Geometry: final body of the model. Coordinates: model frame, mm. Face numbers are marked on the shaded views. Coordinates: 2 decimals unless noted, no trailing zeros. Write each loop counter-clockwise with the first axis right and the second up, starting at its lowest first coordinate (ties: lowest second). Pieces come first, ordered by that corner, then holes. Notation, with made-up numbers: (-38, -3) - (-3, -3) arc R18 cw to (-3, 24) - close; hole circle Ø1 at (23.25, 78). An arc over 180 degrees is marked (long way). Answer as a JSON object with one key per item and string values. Group by question number.
Item 1: Section C-C on x = 52.5. Return loops of the section in (y, z) (3 decimals).
Item 2: Mould query, pull axis X, two halves, no side actions, for the marked faces 1 and 2. Classes: pulls with the +X half, pulls with the -X half, needs draft (parallel to the pull), parting line crosses it, or undercut.
Item 3: First-contact query: pin 1 Ø22.5 at (x, y) = (-52.5, -40) entering from +Z; pin 2 Ø14 at (x, y) = (52.5, 40) entering from +Z. Flat tips, straight axial feed; report the tip coordinate or a pass-through.
Item 4: Section B-B on y = -40. Return loops of the section in (x, z) (3 decimals), and give its area (4 significant figures).
Item 5: Line query: line 1 along Y through (x, z) = (-52.5, 3.75) (3 decimals); line 2 along Y through (x, z) = (55, 6.75); line 3 along X through (y, z) = (-41.5, 9). Output: solid intervals per line, ascending. Write a range as from..to.
Item 6: Section A-A on z = 1.5. Return loops of the section in (x, y) (3 decimals).
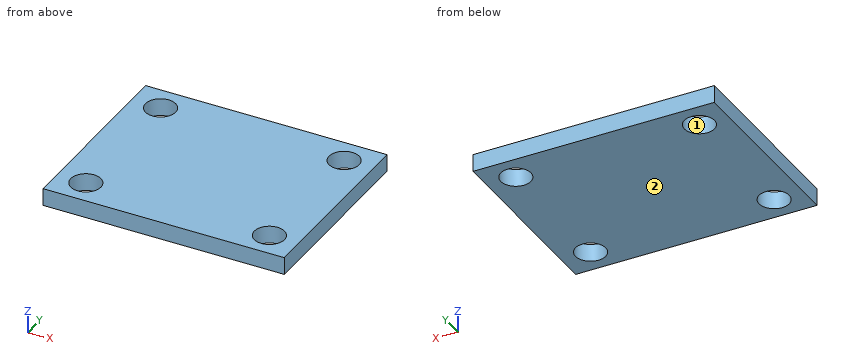
```python
from build123d import *

# Parameters (mm, degrees)
F0_W           = 138
F0_H           = 110
F0_R           = 5
F1_DEPTH       = 10
F2_D           = 11
F2_CBORE_D     = 17.25
F2_CBORE_DEPTH = 10


with BuildPart() as f1:
    # F0 (on Top) → F1 (new body)
    with BuildSketch(Plane.XY):
        Rectangle(F0_W, F0_H)
        with Locations((-52.5, -40)):
            Circle(F0_R, mode=Mode.SUBTRACT)
        with Locations((52.5, -40)):
            Circle(F0_R, mode=Mode.SUBTRACT)
        with Locations((-52.5, 40)):
            Circle(F0_R, mode=Mode.SUBTRACT)
        with Locations((52.5, 40)):
            Circle(F0_R, mode=Mode.SUBTRACT)
        with Locations((52.5, -40)):
            Circle(F0_R)
        with Locations((-52.5, 40)):
            Circle(F0_R)
        with Locations((-52.5, -40)):
            Circle(F0_R)
        with Locations((52.5, 40)):
            Circle(F0_R)
    extrude(amount=F1_DEPTH)

    # F2 (through all)
    with Locations(Plane(origin=(0, 0, 0), x_dir=(1, 0, 0), z_dir=(0, 0, -1))):
        with Locations((-52.5, -40), (52.5, -40), (-52.5, 40), (52.5, 40)):
            CounterBoreHole(F2_D / 2, F2_CBORE_D / 2, F2_CBORE_DEPTH)


solid = f1.part
```
Checks:
{
 "1": {"outline": "(-55, 0) - (-48.625, 0) - (-48.625, 10) - (-55, 10) - close; (-31.375, 0) - (31.375, 0) - (31.375, 10) - (-31.375, 10) - close; (48.625, 0) - (55, 0) - (55, 10) - (48.625, 10) - close"},
 "2": {"face 1": "undercut", "face 2": "needs draft"},
 "3": {"pin 1": "z = 10", "pin 2": "through"},
 "4": {"outline": "(-69, 0) - (-61.125, 0) - (-61.125, 10) - (-69, 10) - close; (-43.875, 0) - (43.875, 0) - (43.875, 10) - (-43.875, 10) - close; (61.125, 0) - (69, 0) - (69, 10) - (61.125, 10) - close", "area": "1,035 mm^2"},
 "5": {"line 1": "-55..-48.625, -31.375..31.375, 48.625..55", "line 2": "-55..-48.25, -31.75..31.75, 48.25..55", "line 3": "-69..-60.99, -44.01..44.01, 60.99..69"},
 "6": {"outline": "(-69, -55) - (69, -55) - (69, 55) - (-69, 55) - close; hole circle Ø17.25 at (-52.5, -40); hole circle Ø17.25 at (-52.5, 40); hole circle Ø17.25 at (52.5, -40); hole circle Ø17.25 at (52.5, 40)"}
}
